Geometry check sheet. Reference: the model listing, model coordinates, mm. A direction names the side the tool comes from. Round coordinates to 2 decimals unless told otherwise and drop trailing zeros. Answer as CSV lines item,"result". Start each with the question number.
```python
from build123d import *


with BuildPart() as part:
    # Sketch1 → Revolve1 (revolve)
    with BuildSketch(Plane(origin=(0, 0, 0), x_dir=(0, 0, -1), z_dir=(1, 0, 0)), mode=Mode.PRIVATE) as revolve1_sk:
        with BuildLine():
            Line((217.594560556, -10), (215.594560556, -10))
            Line((215.594560556, -10), (215.594560556, -12))
            Line((215.594560556, -12), (221.437329759, -12))
            Line((221.437329759, -12), (226.035038621, -13.964961379))
            ThreePointArc((226.035038621, -13.964961379), (240, 0), (226.035038621, 13.964961379))
            Line((226.035038621, 13.964961379), (221.437329759, 12))
            Line((221.437329759, 12), (215.594560556, 12))
            Line((215.594560556, 12), (215.594560556, 10))
            Line((215.594560556, 10), (217.594560556, 10))
            Line((217.594560556, 10), (221.846794436, 10))
            Line((221.846794436, 10), (226.42930017, 11.958463891))
            ThreePointArc((226.42930017, 11.958463891), (238, 0), (226.42930017, -11.958463891))
            Line((226.42930017, -11.958463891), (221.846794436, -10))
            Line((221.846794436, -10), (217.594560556, -10))
        make_face()
    revolve(revolve1_sk.sketch.rotate(Axis((0, 21.897389464, 0), (0, -1, 0)), 180), axis=Axis((0, 21.897389464, 0), (0, -1, 0)))


solid = part.part
```
1. Access from +Z, -Z, +X, -X, +Y, -Y to the whole of each face (thin tool, end or side, straight path). Record for faces 1 (the face through (216.789, -10.095, -48.14)), 2 (the face through (210.468, -11.014, -46.737)), 3 (the face through (48, -12, -212)), 4 (the face through (212, 12, 48)).
2. Thickness scan on probe 1 along Y at (x, z) = (202.5, 79); probe 2 along X at (y, z) = (-10.55, 0); probe 3 along X at (y, z) = (10.7, 0). Record the ranges inside material, lowest first.
3. Go/stop test with flat-tipped pins: pin 1 Ø6 at (y, z) = (-1.5, 145) entering from +X; pin 2 Ø8 at (y, z) = (6.5, -52.5) entering from -X; pin 3 Ø8 at (x, y) = (107.5, -9) entering from -Z. Record where each tip stops, or that it passes through.
Numbers:
1,face 1,"none"
1,face 2,"+Y, -Y"
1,face 3,"-Y"
1,face 4,"+Y"
2,probe 1,"y = -12 to -10, 10 to 12"
2,probe 2,"x = -235.18 to -231.68, -223.13 to -215.59, 215.59 to 223.13, 231.68 to 235.18"
2,probe 3,"x = -235.01 to -231.39, -223.48 to -215.59, 215.59 to 223.48, 231.39 to 235.01"
3,pin 1,"stops at x = 193.41"
3,pin 2,"stops at x = -234.31"
3,pin 3,"stops at z = -214.38"
